from build123d import *

# Parameters (mm, degrees)
F0_R     = 57.5961395205
F1_DEPTH = 25.4
F2_R     = 41.9082998656
F3_DEPTH = 178
F4_R     = 11.649028694
F5_DEPTH = 12.7


# Not quite as in the source:
# - an extrude ends at something that could not be found from the text; its depth is read off the source's solid


with BuildPart() as f1:
    # F0 (on Top) → F1 (new body)
    with BuildSketch(Plane.XY):
        Circle(F0_R)
    extrude(amount=F1_DEPTH)

    # F2 (on Top) → F3 (cut, through all)
    with BuildSketch(Plane.XY):
        Circle(F2_R)
    extrude(amount=-F3_DEPTH, mode=Mode.SUBTRACT)

    # F4 (on Front) → F5 (cut)
    with BuildSketch(Plane.XZ):
        with Locations((-8.324730893, 12.7451797782)):
            Circle(F4_R)
    extrude(amount=-F5_DEPTH, mode=Mode.SUBTRACT)


solid = f1.part
Geometry: final body of the model. Coordinates: model frame, mm. A direction names the side the tool comes from. Give positions to 0.01 mm unless a question says otherwise; leave off trailing zeros. Order: outer loops, then holes, each group sorted by start corner. A loop starts at its lowest first (then second) coordinate and runs counter-clockwise, first axis right, second up. Notation, with made-up numbers: (25.25, 47.5) -> (68.25, 47.5) arc R26 cw to (68.25, 84.5) -> close; hole circle Ø7 at (-19.75, 29.25). An arc over 180 degrees is marked (long way). Write each question's results on one line, items separated by ' | '.
1) Cut plane B-B (z = 10.25). Output: boundary loops of the cut face in (x, y), and give its area (3 significant figures).
Geometry says:
outline: circle Ø115.19 at (0, 0); hole (-19.7, 0) -> (3.05, 0) -> (3.05, 12.7) -> (-19.7, 12.7) -> close | area: 10,100 mm²
2) Line query: line 1 along Y through (x, z) = (1.5, 18.75); line 2 along Y through (x, z) = (-8, 20); line 3 along X through (y, z) = (3, 2.5). Output: solid intervals per line, ascending.
Geometry says:
line 1: y = -57.58 to 0, 12.7 to 57.58 | line 2: y = -57.04 to 0, 12.7 to 57.04 | line 3: x = -57.52 to -13.87, -2.78 to 57.52
3) First-contact query: pin 1 Ø12 at (y, z) = (-45.5, 20.5) entering from -X; pin 2 Ø2 at (x, z) = (13, 19.5) entering from +Y; pin 3 Ø4 at (y, z) = (-40.5, 20) entering from -X. Flat tips, straight axial feed; report the tip coordinate or a pass-through.
Geometry says:
pin 1: stops at x = -41.92 | pin 2: stops at y = 56.33 | pin 3: stops at x = -42.84
4) Set-up query: faces 4 (the face through (-1, 1, 25.4)), 5 (the face through (-17.6, 6.3, 5.7)). Return all of +Z, -Z, +X, -X, +Y, -Y with unobstructed straight access to the full face (end or side cutting, diameter ignored); none if empty.
Geometry says:
face 4: +Z, +X, -X, +Y, -Y | face 5: none
5) Cut plane A-A (x = -1). Output: boundary loops of the cut face in (y, z).
Geometry says:
outline: (-57.59, 0) -> (57.59, 0) -> (57.59, 25.4) -> (-57.59, 25.4) -> close; hole (0, 3.69) -> (12.7, 3.69) -> (12.7, 21.8) -> (0, 21.8) -> close
6) Cut plane C-C (y = -27). Output: boundary loops of the cut face in (x, z).
Geometry says:
outline: (-50.88, 0) -> (50.88, 0) -> (50.88, 25.4) -> (-50.88, 25.4) -> close
7) Draft query along Y for faces 1 (the face through (54.936, 17.3, 12.522)), 2 (the face through (-8, 12.7, 13)), 3 (the face through (-1, 1, 0)). Return one class per face: released by +Y, released by -Y, zero draft, split by the parting line, or undercut.
Geometry says:
face 1: split by the parting line | face 2: undercut | face 3: zero draft
8) Cut plane D-D (z = 22). Output: boundary loops of the cut face in (x, y).
Geometry says:
outline: circle Ø115.19 at (0, 0); hole (-15.4, 0) -> (-1.25, 0) -> (-1.25, 12.7) -> (-15.4, 12.7) -> close
